```python
from build123d import *

# Parameters (mm, degrees)
SKETCH_1_R          = 1.15
EXTRUDE_1_DEPTH     = 2
FILLET_1_R          = 3
SKETCH_2_R          = 1.15
CUT_EXTRUDE_1_DEPTH = 2
SKETCH_3_W          = 9
SKETCH_3_H          = 30
CUT_EXTRUDE_2_DEPTH = 2
CUT_EXTRUDE_3_DEPTH = 3


with BuildPart() as part:
    # 草图1 → 凸台-拉伸1 (new body)
    with BuildSketch(Plane(origin=(0, 0, 0), x_dir=(1, 0, 0), z_dir=(0, 1, 0))):
        Polygon((64, -39), (5, -39), (5, -3), (-4, -3), (-4, 21), (5, 21), (5, 43), (64, 43), align=None)
        Circle(SKETCH_1_R, mode=Mode.SUBTRACT)
        with Locations((0, 18)):
            Circle(SKETCH_1_R, mode=Mode.SUBTRACT)
    extrude(amount=EXTRUDE_1_DEPTH)

    # 圆角1
    fillet_1_edges = [part.edges().sort_by_distance(p)[0] for p in [
        (5, 1, -43),
        (64, 1, -43),
        (64, 1, 39),
        (5, 1, 39),
        (5, 1, 3),
        (-4, 1, 3),
        (-4, 1, -21),
        (5, 1, -21),
    ]]
    fillet(fillet_1_edges, radius=FILLET_1_R)

    # 草图2 → 切除-拉伸1 (cut)
    with BuildSketch(Plane(origin=(0, 2, 0), x_dir=(1, 0, 0), z_dir=(0, 1, 0))):
        with Locations((10, 18)):
            Circle(SKETCH_2_R)
        with Locations((10, 0)):
            Circle(SKETCH_2_R)
    extrude(amount=-CUT_EXTRUDE_1_DEPTH, mode=Mode.SUBTRACT)

    # 草图3 → 切除-拉伸2 (cut)
    with BuildSketch(Plane(origin=(0, 2, 0), x_dir=(1, 0, 0), z_dir=(0, 1, 0))):
        with Locations((0.5, 9)):
            Rectangle(SKETCH_3_W, SKETCH_3_H)
    extrude(amount=-CUT_EXTRUDE_2_DEPTH, mode=Mode.SUBTRACT)

    # 草图4 → 切除-拉伸3 (cut, through all)
    with BuildSketch(Plane(origin=(0, 2, 0), x_dir=(1, 0, 0), z_dir=(0, 1, 0))):
        with BuildLine():
            Line((24, 39), (54, 39))
            ThreePointArc((54, 39), (56, 37), (54, 35))
            Line((54, 35), (24, 35))
            ThreePointArc((24, 35), (22, 37), (24, 39))
        make_face()
        with BuildLine():
            Line((24, 29), (54, 29))
            ThreePointArc((54, 29), (56, 27), (54, 25))
            Line((54, 25), (24, 25))
            ThreePointArc((24, 25), (22, 27), (24, 29))
        make_face()
        with BuildLine():
            Line((24, 19), (54, 19))
            ThreePointArc((54, 19), (56, 17), (54, 15))
            Line((54, 15), (24, 15))
            ThreePointArc((24, 15), (22, 17), (24, 19))
        make_face()
        with BuildLine():
            Line((24, 9), (54, 9))
            ThreePointArc((54, 9), (56, 7), (54, 5))
            Line((54, 5), (24, 5))
            ThreePointArc((24, 5), (22, 7), (24, 9))
        make_face()
        with BuildLine():
            Line((24, -1), (54, -1))
            ThreePointArc((54, -1), (56, -3), (54, -5))
            Line((54, -5), (24, -5))
            ThreePointArc((24, -5), (22, -3), (24, -1))
        make_face()
        with BuildLine():
            Line((24, -11), (54, -11))
            ThreePointArc((54, -11), (56, -13), (54, -15))
            Line((54, -15), (24, -15))
            ThreePointArc((24, -15), (22, -13), (24, -11))
        make_face()
        with BuildLine():
            Line((24, -21), (54, -21))
            ThreePointArc((54, -21), (56, -23), (54, -25))
            Line((54, -25), (24, -25))
            ThreePointArc((24, -25), (22, -23), (24, -21))
        make_face()
        with BuildLine():
            Line((24, -31), (54, -31))
            ThreePointArc((54, -31), (56, -33), (54, -35))
            Line((54, -35), (24, -35))
            ThreePointArc((24, -35), (22, -33), (24, -31))
        make_face()
    extrude(amount=-CUT_EXTRUDE_3_DEPTH, mode=Mode.SUBTRACT)


solid = part.part
```
Here's how the part is built. I have some questions about the finished solid (model axes, mm). Give positions to 0.01 mm unless a question says otherwise; leave off trailing zeros. Order: outer loops, then holes, each group sorted by start corner. A loop starts at its lowest first (then second) coordinate and runs counter-clockwise, first axis right, second up. Notation, with made-up numbers: M 57.25,31.5 L 73.25,31.5 A9 cw 73.25,36.5 Z; hole C 35,74.5 d5. An arc over 180 degrees is marked long. Use a Markdown table: item, result. Add a question column.
1. I need wall thicknesses on probe 1 along Z at (x, y) = (10, 0.8); probe 2 along X at (y, z) = (0.85, -18); probe 3 along Z at (x, y) = (9, 1.3). Which ranges of each line are inside material? Lowest first, please. Write a range as from..to.
2. Suppose I cut it at B-B (x = 32.5). Give the number of separate pieces and of enclosed holes in the cut face, and give its area (3 significant figures).
3. Suppose I cut it at A-A (z = 0). List the corners of the cut face in (x, y) for me, and give its area (3 significant figures).
4. If we mould it in two halves opening along Z, with no side actions, what happens to faces 1 (the flat face through (34, 1, -43)), 2 (the cylindrical face through (22, 1, -17)), 3 (the flat face through (39, 1, -39))? For each: +Z half, -Z half, draft (parallel to the pull), parting line (faces both ways), or undercut.
5. Suppose I cut it at C-C (z = 33). List the corners of the cut face in (x, y) for me, and give its area (3 significant figures).
Results list:
| question | item | result |
|---|---|---|
| 1 | probe 1 | z = -43..-19.15, -16.85..-1.15, 1.15..39 |
| 1 | probe 2 | x = 5..8.85, 11.15..22.27, 55.73..64 |
| 1 | probe 3 | z = -43..-18.57, -17.43..-0.57, 0.57..39 |
| 2 | separate pieces | 9 |
| 2 | enclosed holes | 0 |
| 2 | area | 100 mm² |
| 3 | outline | M 5,0 L 8.85,0 L 8.85,2 L 5,2 Z; M 11.15,0 L 64,0 L 64,2 L 11.15,2 Z |
| 3 | area | 113 mm² |
| 4 | face 1 | -Z half |
| 4 | face 2 | undercut |
| 4 | face 3 | undercut |
| 5 | outline | M 5,0 L 22,0 L 22,2 L 5,2 Z; M 56,0 L 64,0 L 64,2 L 56,2 Z |
| 5 | area | 50.0 mm² |
